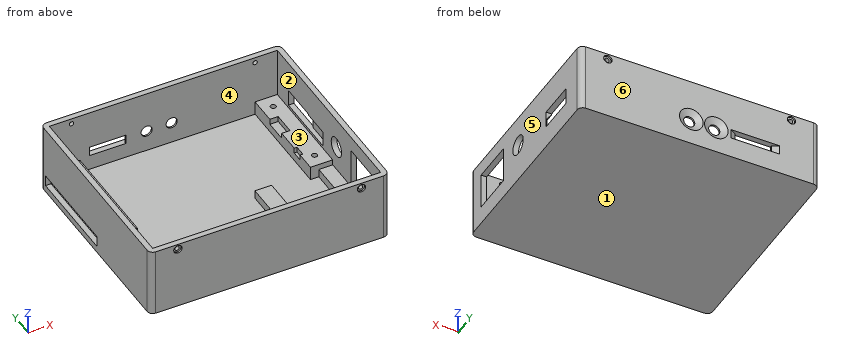
```python
from build123d import *
from OCP.BRepFilletAPI import BRepFilletAPI_MakeChamfer

# Parameters (mm, degrees)
SKETCH1_W           = 86
SKETCH1_H           = 74
BOSS_EXTRUDE1_DEPTH = 25
SKETCH3_W           = 82
SKETCH3_H           = 70
CUT_EXTRUDE1_DEPTH  = 23
SKETCH4_W           = 8
SKETCH4_H           = 37.5
SKETCH4_W_2         = 1.4
BOSS_EXTRUDE2_DEPTH = 5
SKETCH5_W           = 3
SKETCH5_H           = 8
SKETCH5_W_2         = 1
SKETCH5_H_2         = 4
CUT_EXTRUDE2_DEPTH  = 2
SKETCH6_R           = 1
CUT_EXTRUDE3_DEPTH  = 5
SKETCH7_W           = 4
SKETCH7_H           = 35
CUT_EXTRUDE4_DEPTH  = 5
SKETCH8_W           = 6
SKETCH8_H           = 23.5
CUT_EXTRUDE5_DEPTH  = 5
SKETCH9_W           = 5
SKETCH9_H           = 32.5
SKETCH9_W_2         = 6
BOSS_EXTRUDE3_DEPTH = 3
SKETCH10_R          = 0.9
CUT_EXTRUDE6_DEPTH  = 4
SKETCH11_W          = 13
SKETCH11_H          = 15
CUT_EXTRUDE7_DEPTH  = 4
FILLET1_R           = 2
SKETCH12_R          = 3.5
CUT_EXTRUDE8_DEPTH  = 4
SKETCH13_R          = 2
SKETCH13_W          = 13
SKETCH13_H          = 3.4
CUT_EXTRUDE9_DEPTH  = 4
CHAMFER1_SIZE       = 1.4
CHAMFER1_SIZE2      = 2.240468341
SKETCH14_R          = 0.8
CUT_EXTRUDE10_DEPTH = 76
SKETCH15_R          = 1.5
CUT_EXTRUDE11_DEPTH = 0.6
CUT_EXTRUDE12_START = -0.6
SKETCH16_R          = 1.5
CUT_EXTRUDE12_DEPTH = 0.6
SKETCH17_W          = 2
SKETCH17_H          = 10
BOSS_EXTRUDE4_DEPTH = 2.4
SKETCH18_W          = 3.6
SKETCH18_H          = 10
BOSS_EXTRUDE5_DEPTH = 0.4
CHAMFER2_SIZE       = 2
CHAMFER2_SIZE2      = 1.562571253
SKETCH20_W          = 11
SKETCH20_H          = 1.4
BOSS_EXTRUDE6_DEPTH = 5


with BuildPart() as part:
    # Sketch1 → Boss-Extrude1 (new body)
    with BuildSketch(Plane.XY):
        with Locations((43, 37)):
            Rectangle(SKETCH1_W, SKETCH1_H)
    extrude(amount=BOSS_EXTRUDE1_DEPTH)

    # Sketch3 → Cut-Extrude1 (cut)
    with BuildSketch(Plane.XY.offset(25)):
        with Locations((43, 37)):
            Rectangle(SKETCH3_W, SKETCH3_H)
    extrude(amount=-CUT_EXTRUDE1_DEPTH, mode=Mode.SUBTRACT)

    # Sketch4 → Boss-Extrude2 (add)
    with BuildSketch(Plane.XY.offset(2)):
        with Locations((80, 53.25)):
            Rectangle(SKETCH4_W, SKETCH4_H)
        with Locations((12.3, 53.25)):
            Rectangle(SKETCH4_W_2, SKETCH4_H)
    extrude(amount=BOSS_EXTRUDE2_DEPTH)

    # Sketch5 → Cut-Extrude2 (cut)
    with BuildSketch(Plane.XY.offset(7)):
        with Locations((77.5, 58)):
            Rectangle(SKETCH5_W, SKETCH5_H)
        with Locations((76.5, 43.5)):
            Rectangle(SKETCH5_W_2, SKETCH5_H_2)
    extrude(amount=-CUT_EXTRUDE2_DEPTH, mode=Mode.SUBTRACT)

    # Sketch6 → Cut-Extrude3 (cut)
    with BuildSketch(Plane.XY.offset(7)):
        with Locations((80, 67.25)):
            Circle(SKETCH6_R)
        with Locations((80, 39.25)):
            Circle(SKETCH6_R)
    extrude(amount=-CUT_EXTRUDE3_DEPTH, mode=Mode.SUBTRACT)

    # Sketch7 → Cut-Extrude4 (cut)
    with BuildSketch(Plane(origin=(2, 0, 0), x_dir=(0, 0, -1), z_dir=(1, 0, 0))):
        with Locations((-4.4, 53.35)):
            Rectangle(SKETCH7_W, SKETCH7_H)
    extrude(amount=-CUT_EXTRUDE4_DEPTH, mode=Mode.SUBTRACT)

    # Sketch8 → Cut-Extrude5 (cut)
    with BuildSketch(Plane.ZY.offset(-84)):
        with Locations((11, 52.75)):
            Rectangle(SKETCH8_W, SKETCH8_H)
    extrude(amount=-CUT_EXTRUDE5_DEPTH, mode=Mode.SUBTRACT)

    # Sketch9 → Boss-Extrude3 (add)
    with BuildSketch(Plane.XY.offset(2)):
        with Locations((81.5, 18.25)):
            Rectangle(SKETCH9_W, SKETCH9_H)
        with Locations((59, 18.25)):
            Rectangle(SKETCH9_W_2, SKETCH9_H)
    extrude(amount=BOSS_EXTRUDE3_DEPTH)

    # Sketch10 → Cut-Extrude6 (cut)
    with BuildSketch(Plane.XY.offset(5)):
        with Locations((59, 13.5)):
            Circle(SKETCH10_R)
    extrude(amount=-CUT_EXTRUDE6_DEPTH, mode=Mode.SUBTRACT)

    # Sketch11 → Cut-Extrude7 (cut)
    with BuildSketch(Plane.ZY.offset(-84)):
        with Locations((13.1, 14.5)):
            Rectangle(SKETCH11_W, SKETCH11_H)
    extrude(amount=-CUT_EXTRUDE7_DEPTH, mode=Mode.SUBTRACT)

    # Fillet1
    fillet1_edges = [part.edges().sort_by_distance(p)[0] for p in [
        (0, 74, 12.5),
        (86, 74, 12.5),
        (86, 0, 12.5),
        (0, 0, 12.5),
    ]]
    fillet(fillet1_edges, radius=FILLET1_R)

    # Sketch12 → Cut-Extrude8 (cut)
    with BuildSketch(Plane.ZY.offset(-84)):
        with Locations(Location((14, 32, 0), (0, 0, 270))):
            Circle(SKETCH12_R)
    extrude(amount=-CUT_EXTRUDE8_DEPTH, mode=Mode.SUBTRACT)

    # Sketch13 → Cut-Extrude9 (cut)
    with BuildSketch(Plane(origin=(0, 72, 0), x_dir=(-1, 0, 0), z_dir=(0, -1, 0))):
        with Locations(Location((-37, -9.8, 0), (0, 0, 90))):
            Circle(SKETCH13_R)
        with Locations(Location((-46, -9.8, 0), (0, 0, 90))):
            Circle(SKETCH13_R)
        with Locations((-23, -9.3)):
            Rectangle(SKETCH13_W, SKETCH13_H)
    extrude(amount=-CUT_EXTRUDE9_DEPTH, mode=Mode.SUBTRACT)

    # Chamfer1: one chamfer whose edges measure the first distance from different faces: ONE call of the kernel's chamfer builder (chamfer() names one face for all edges)
    chamfer1_edges_1 = [part.edges().sort_by_distance(p)[0] for p in [
        (16.5, 74, 9.3),
    ]]
    chamfer1_side_1 = [part.faces().sort_by_distance(p)[0] for p in [
        (16.5, 73, 9.3),
    ]]
    chamfer1_edges_2 = [part.edges().sort_by_distance(p)[0] for p in [
        (29.5, 74, 9.3),
    ]]
    chamfer1_side_2 = [part.faces().sort_by_distance(p)[0] for p in [
        (29.5, 73, 9.3),
    ]]
    chamfer1_edges_3 = [part.edges().sort_by_distance(p)[0] for p in [
        (37, 74, 11.8),
    ]]
    chamfer1_side_3 = [part.faces().sort_by_distance(p)[0] for p in [
        (37, 73, 11.8),
    ]]
    chamfer1_edges_4 = [part.edges().sort_by_distance(p)[0] for p in [
        (46, 74, 11.8),
    ]]
    chamfer1_side_4 = [part.faces().sort_by_distance(p)[0] for p in [
        (46, 73, 11.8),
    ]]
    chamfer1 = BRepFilletAPI_MakeChamfer(part.part.solid().wrapped)
    for e in chamfer1_edges_1:
        chamfer1.Add(CHAMFER1_SIZE, CHAMFER1_SIZE2, e.wrapped, chamfer1_side_1[0].wrapped)  # the first distance lies on this face
    for e in chamfer1_edges_2:
        chamfer1.Add(CHAMFER1_SIZE, CHAMFER1_SIZE2, e.wrapped, chamfer1_side_2[0].wrapped)  # the first distance lies on this face
    for e in chamfer1_edges_3:
        chamfer1.Add(CHAMFER1_SIZE, CHAMFER1_SIZE2, e.wrapped, chamfer1_side_3[0].wrapped)  # the first distance lies on this face
    for e in chamfer1_edges_4:
        chamfer1.Add(CHAMFER1_SIZE, CHAMFER1_SIZE2, e.wrapped, chamfer1_side_4[0].wrapped)  # the first distance lies on this face
    add(Compound.cast(chamfer1.Shape()), mode=Mode.REPLACE)

    # Sketch14 → Cut-Extrude10 (cut)
    with BuildSketch(Plane(origin=(0, 0, 0), x_dir=(-1, 0, 0), z_dir=(0, -1, 0))):
        with Locations(Location((-10, -23, 0), (0, 0, 90))):
            Circle(SKETCH14_R)
        with Locations(Location((-76, -23, 0), (0, 0, 90))):
            Circle(SKETCH14_R)
    extrude(amount=-CUT_EXTRUDE10_DEPTH, mode=Mode.SUBTRACT)

    # Sketch15 → Cut-Extrude11 (cut)
    with BuildSketch(Plane(origin=(0, 0, 0), x_dir=(-1, 0, 0), z_dir=(0, -1, 0))):
        with Locations(Location((-10, -23, 0), (0, 0, 90))):
            Circle(SKETCH15_R)
        with Locations(Location((-76, -23, 0), (0, 0, 90))):
            Circle(SKETCH15_R)
    extrude(amount=-CUT_EXTRUDE11_DEPTH, mode=Mode.SUBTRACT)

    # Sketch16 → Cut-Extrude12 (cut)
    with BuildSketch(Plane(origin=(0, 74, 0), x_dir=(1, 0, 0), z_dir=(0, 1, 0)).offset(CUT_EXTRUDE12_START)):
        with Locations(Location((76, -23, 0), (0, 0, 90))):
            Circle(SKETCH16_R)
        with Locations(Location((10, -23, 0), (0, 0, 90))):
            Circle(SKETCH16_R)
    extrude(amount=CUT_EXTRUDE12_DEPTH, mode=Mode.SUBTRACT)

    # Sketch17 → Boss-Extrude4 (add)
    with BuildSketch(Plane(origin=(0, 0, 14), x_dir=(-1, 0, 0), z_dir=(0, 0, -1))):
        with Locations((-85, 46)):
            Rectangle(SKETCH17_W, SKETCH17_H)
    extrude(amount=BOSS_EXTRUDE4_DEPTH)

    # Sketch18 → Boss-Extrude5 (add)
    with BuildSketch(Plane(origin=(86, 0, 0), x_dir=(0, 0, -1), z_dir=(1, 0, 0))):
        with Locations((-9.8, 46)):
            Rectangle(SKETCH18_W, SKETCH18_H)
    extrude(amount=-BOSS_EXTRUDE5_DEPTH)

    # Chamfer2
    chamfer2_edges = [part.edges().sort_by_distance(p)[0] for p in [
        (84, 46, 11.6),
    ]]
    chamfer2_side = [part.faces().sort_by_distance(p)[0] for p in [
        (84, 38.391894294, 16.636900107),
    ]]
    chamfer(chamfer2_edges, length=CHAMFER2_SIZE, length2=CHAMFER2_SIZE2, reference=chamfer2_side[0])

    # Sketch20 → Boss-Extrude6 (add)
    with BuildSketch(Plane.XY.offset(2)):
        with Locations((7.5, 33.8)):
            Rectangle(SKETCH20_W, SKETCH20_H)
    extrude(amount=BOSS_EXTRUDE6_DEPTH)


solid = part.part
```
For this review, take the finished solid that the model builds, in its own axes (mm). Face numbers are marked on the shaded views. A direction names the side the tool comes from. Coordinates: 2 decimals unless noted, no trailing zeros. Loops run counter-clockwise (first coordinate to the right, second up) from the corner with the lowest first, then second, coordinate; pieces in that order, holes last. Notation, with made-up numbers: (15, -31.75) -> (43, -31.75) arc R31 cw to (43, -4.75) -> close; hole circle Ø4 at (42.25, 23.5). An arc over 180 degrees is marked (long way). Return JSON: item names as keys, results as strings. Group by question number.
(1) For pin 1 Ø2.5 at (x, z) = (10, 23) entering from +Y; pin 2 Ø0.5 at (x, z) = (84.5, 11.5) entering from +Y; pin 3 Ø2 at (x, y) = (79.5, 67.5) entering from +Z, all flat-tipped, find the tip position at first contact; note any pin that passes through.
(2) Consider section C-C, the plane z = 18.5. Give the boundary of the cut face in (x, y), plus the area to 3 significant figures.
(3) Mouldability with a two-part tool opening along X and no side actions: class the marked faces 3, 4, 5 and 6 as pulls with the +X half, pulls with the -X half, needs draft (parallel to the pull), parting line crosses it, or undercut.
(4) Tool access review of the marked faces 1 and 2: name each direction out of +Z, -Z, +X, -X, +Y, -Y from which nothing blocks a thin tool from reaching the whole face with its end or side.
(5) Consider section A-A, the plane y = 59. Give the boundary of the cut face in (x, z).
(6) To check wall thickness, follow L1, parallel to Y at x = 8.5, z = 5.5; L2, parallel to X at y = 1.7, z = 23; L3, parallel to Y at x = 25.5, z = 12.5. State the ranges of each line that lie inside material, in increasing order.
(7) Consider section B-B, the plane x = 37. Give the boundary of the cut face in (y, z).
Results below:
{
 "1": {"pin 1": "stops at y = 73.4", "pin 2": "stops at y = 73.98", "pin 3": "stops at z = 7"},
 "2": {"outline": "(0, 2) arc R2 ccw to (2, 0) -> (84, 0) arc R2 ccw to (86, 2) -> (86, 7) -> (84, 7) -> (84, 2) -> (2, 2) -> (2, 72) -> (84, 72) -> (84, 22) -> (86, 22) -> (86, 72) arc R2 ccw to (84, 74) -> (2, 74) arc R2 ccw to (0, 72) -> close", "area": "591 mm2"},
 "3": {"face 3": "undercut", "face 4": "undercut", "face 5": "pulls with the +X half", "face 6": "needs draft"},
 "4": {"face 1": "-Z, +X, -X, +Y, -Y", "face 2": "+Z"},
 "5": {"outline": "(0, 0) -> (86, 0) -> (86, 8) -> (84, 8) -> (84, 7) -> (79, 7) -> (79, 5) -> (76, 5) -> (76, 2) -> (13, 2) -> (13, 7) -> (11.6, 7) -> (11.6, 2) -> (2, 2) -> (2, 2.4) -> (0, 2.4) -> close; (0, 6.4) -> (2, 6.4) -> (2, 25) -> (0, 25) -> close; (84, 14) -> (86, 14) -> (86, 25) -> (84, 25) -> close"},
 "6": {"L1": "y = 0 to 2, 33.1 to 34.5, 72 to 74", "L2": "x = 0.02 to 9.2, 10.8 to 75.2, 76.8 to 85.98", "L3": "y = 0 to 2, 72 to 74"},
 "7": {"outline": "(0, 0) -> (74, 0) -> (74, 5.56) -> (72.6, 7.8) -> (72, 7.8) -> (72, 2) -> (2, 2) -> (2, 25) -> (0, 25) -> close; (72, 11.8) -> (72.6, 11.8) -> (74, 14.04) -> (74, 25) -> (72, 25) -> close"}
}
